Read the model definition and answer for the solid it produces. Units are mm, in the model's axes. A direction names the side the tool comes from. Coordinates: 2 decimals unless noted, no trailing zeros. Write each loop counter-clockwise with the first axis right and the second up, starting at its lowest first coordinate (ties: lowest second). Pieces come first, ordered by that corner, then holes.
(1) Given pin 1 (0.8 mm diameter, centred on x = 11, y = 5.5, fed in from +Z); pin 2 (3.5 mm diameter, centred on x = 12, z = -8, fed in from -Y); pin 3 (2 mm diameter, centred on y = 8.5, z = -11.5, fed in from +X), each flat-ended and moving along its own axis, determine where each tip first touches the part or whether it passes through.
(2) Which of the six approach directions +Z, -Z, +X, -X, +Y, -Y give full straight-line access (tool end or side, diameter ignored) to faces 3 (the cylindrical face through (17.845, 9.014, -8.921)), 4 (the flat face through (12, 6, -8)), 5 (the flat face through (5, 7, -8))?
(3) The part is cut by section C-C, the plane z = -13.25. Determine the outline of the cut face in (x, y).
(4) Determine the mould class of faces 1 (the flat face through (18, 5, -14)), 2 (the cylindrical face through (14.808, 9.699, -13.285)) for opening direction Z: pulls with the +Z half, pulls with the -Z half, needs draft (parallel to the pull), parting line crosses it, or undercut.
(5) The part is cut by section A-A, the plane x = 18.5. Determine the outline of the cut face in (y, z), and give its area (3 significant figures).
(6) The part is cut by section B-B, the plane x = 12. Determine the outline of the cut face in (y, z).
(7) The part is cut by section D-D, the plane y = 6.4. State how many separate pieces and enclosed holes the cut face has, and give its area (3 significant figures).
(8) Straight lines are drawn through the part: line 1 along Z through (x, y) = (10.5, 7.9); line 2 along Z through (x, y) = (12, 5.95); line 3 along Z through (x, y) = (18.25, 7.7). For each, find the intervals that lie inside material, in ascending order.
```python
from build123d import *

# Parameters (mm, degrees)
BOSS_EXTRUDE1_DEPTH = 10
CUT_EXTRUDE3_DEPTH  = 28.676705006
CUT_EXTRUDE6_START  = -13
CUT_EXTRUDE6_DEPTH  = 2
CUT_EXTRUDE14_START = -3
CUT_EXTRUDE14_DEPTH = 2
CUT_EXTRUDE7_START  = 10
SKETCH8_R           = 2.75
CUT_EXTRUDE7_DEPTH  = 2
CUT_EXTRUDE8_START  = -16
SKETCH10_R          = 2.25
CUT_EXTRUDE8_DEPTH  = 3
CUT_EXTRUDE9_DEPTH  = 5
SKETCH18_R          = 0.75
CUT_EXTRUDE12_DEPTH = 28.676705006
CUT_EXTRUDE13_START = 5
SKETCH19_W          = 4
SKETCH19_H          = 4
CUT_EXTRUDE13_DEPTH = 1
CUT_EXTRUDE15_START = -1
SKETCH5_R           = 1.75
CUT_EXTRUDE15_DEPTH = 2
CUT_EXTRUDE16_START = -1
CUT_EXTRUDE16_DEPTH = 2
FILLET2_R           = 0.5
FILLET3_R           = 1
POT_INSERT_DEPTH    = 2.5
POT_START           = 4
SKETCH6_R           = 2.75
POT_HOLE_DEPTH      = 1.5
SCREW_START         = 11
SKETCH14_R          = 0.8
SCREW_HOLES_DEPTH   = 9
SCREW_START_2       = 10
SKETCH15_R          = 1.25
SCREW_HEADS_DEPTH   = 2
SKETCH13_W          = 21
SKETCH13_H          = 15
CUT_EXTRUDE11_DEPTH = 5


with BuildPart() as part:
    # Sketch1 → Boss-Extrude1 (new body)
    with BuildSketch(Plane(origin=(0, 0, 0), x_dir=(1, 0, 0), z_dir=(0, 1, 0))):
        with BuildLine():
            Line((21, 15), (21, 8))
            Line((21, 8), (21, 1))
            Line((21, 1), (12, 1))
            Line((12, 1), (2.253205655, 1))
            ThreePointArc((2.253205655, 1), (0, 8), (2.253205655, 15))
            Line((2.253205655, 15), (12, 15))
            Line((12, 15), (21, 15))
        make_face()
    extrude(amount=BOSS_EXTRUDE1_DEPTH)

    # Sketch4 → Cut-Extrude3 (cut, through all)
    with BuildSketch(Plane.XY):
        with BuildLine():
            Line((21, 14), (12, 14))
            ThreePointArc((12, 14), (18.363961031, 11.363961031), (21, 5))
            Line((21, 5), (21, 14))
        make_face()
        with BuildLine():
            Line((21, -4), (21, 5))
            ThreePointArc((21, 5), (18.363961031, -1.363961031), (12, -4))
            Line((12, -4), (21, -4))
        make_face()
    extrude(amount=-CUT_EXTRUDE3_DEPTH, mode=Mode.SUBTRACT)

    # Sketch7 → Cut-Extrude6 (cut)
    with BuildSketch(Plane.XY.offset(CUT_EXTRUDE6_START)):
        Polygon((21, 5.5), (21, 11), (10, 11), (10, 7.5), (0, 7.5), (0, 3.5), (21, 3.5), align=None)
    extrude(amount=CUT_EXTRUDE6_DEPTH, mode=Mode.SUBTRACT)

    # Sketch21 → Cut-Extrude14 (cut)
    with BuildSketch(Plane.XY.offset(CUT_EXTRUDE14_START)):
        Polygon((21, 5.5), (21, 11), (10, 11), (10, 7.5), (0, 7.5), (0, 3.5), (21, 3.5), align=None)
    extrude(amount=-CUT_EXTRUDE14_DEPTH, mode=Mode.SUBTRACT)

    # Sketch8 → Cut-Extrude7 (cut)
    with BuildSketch(Plane(origin=(0, 0, 0), x_dir=(1, 0, 0), z_dir=(0, 1, 0)).offset(CUT_EXTRUDE7_START)):
        with Locations(Location((12, 8, 0), (0, 0, 270))):
            Circle(SKETCH8_R)
    extrude(amount=-CUT_EXTRUDE7_DEPTH, mode=Mode.SUBTRACT)

    # Sketch10 → Cut-Extrude8 (cut)
    with BuildSketch(Plane.XY.offset(CUT_EXTRUDE8_START)):
        with Locations(Location((12, 5, 0), (0, 0, 221.810314896))):
            Circle(SKETCH10_R)
    extrude(amount=CUT_EXTRUDE8_DEPTH, mode=Mode.SUBTRACT)

    # Sketch11 → Cut-Extrude9 (cut)
    with BuildSketch(Plane(origin=(0, 0, 0), x_dir=(0, 0, -1), z_dir=(1, 0, 0))):
        Polygon((8, 2), (13, 2), (13, 8), (3, 8), (3, 2), align=None)
    extrude(amount=CUT_EXTRUDE9_DEPTH, mode=Mode.SUBTRACT)

    # Sketch18 → Cut-Extrude12 (cut, through all)
    with BuildSketch(Plane.XY):
        with Locations((12, 5)):
            Circle(SKETCH18_R)
    extrude(amount=-CUT_EXTRUDE12_DEPTH, mode=Mode.SUBTRACT)

    # Sketch19 → Cut-Extrude13 (cut, symmetric)
    with BuildSketch(Plane(origin=(0, 0, 0), x_dir=(1, 0, 0), z_dir=(0, 1, 0)).offset(CUT_EXTRUDE13_START)):
        with Locations((12, 8)):
            Rectangle(SKETCH19_W, SKETCH19_H)
    extrude(amount=CUT_EXTRUDE13_DEPTH, both=True, mode=Mode.SUBTRACT)

    # Sketch5 → Cut-Extrude15 (cut)
    with BuildSketch(Plane.XY.offset(CUT_EXTRUDE15_START)):
        with Locations((12, 5)):
            Circle(SKETCH5_R)
    extrude(amount=-CUT_EXTRUDE15_DEPTH, mode=Mode.SUBTRACT)

    # Sketch26 → Cut-Extrude16 (cut)
    with BuildSketch(Plane.XY.offset(CUT_EXTRUDE16_START)):
        with BuildLine():
            Line((16.483314774, 10), (19.483314774, 10))
            ThreePointArc((19.483314774, 10), (20.800790614, 6.883105034), (20.874119675, 3.5))
            Line((20.874119675, 3.5), (17.874119675, 3.5))
            ThreePointArc((17.874119675, 3.5), (17.800790614, 6.883105034), (16.483314774, 10))
        make_face()
    extrude(amount=-CUT_EXTRUDE16_DEPTH, mode=Mode.SUBTRACT)

    # Fillet2
    fillet2_edges = [part.edges().sort_by_distance(p)[0] for p in [
        (12, 8, -10.75),
    ]]
    fillet(fillet2_edges, radius=FILLET2_R)

    # Fillet3
    # the kernel refuses this fillet: 1 mm, written as the material it takes off along each edge
    with BuildSketch(Plane(origin=(12, 5, -13), x_dir=(0.6472427025312245, 0.7622839917118008, 0), z_dir=(-0.7622839917118008, 0.6472427025312245, 0))) as fillet3_piece_1_section:
        with BuildLine():
            CenterArc((9 - FILLET3_R, FILLET3_R), FILLET3_R, 270, 90)
            Line((9 - FILLET3_R, 0), (9, 0))
            Line((9, 0), (9, FILLET3_R))
        make_face()
    fillet3_piece_1 = revolve(axis=Axis((12, 5, -13), (0, 0, -1)), revolution_arc=75.177010416, mode=Mode.PRIVATE)
    fillet3_piece_1 = split(fillet3_piece_1, bisect_by=Plane(origin=(20.22008164, 3.5, -13.28352735), z_dir=(0, 1, 0)), keep=Keep.TOP, mode=Mode.PRIVATE)
    add(fillet3_piece_1, mode=Mode.SUBTRACT)
    with BuildSketch(Plane(origin=(12, 5, -11), x_dir=(0.9025022770828605, -0.43068508200337235, 0), z_dir=(-0.43068508200337235, -0.9025022770828605, 0))) as fillet3_piece_2_section:
        with BuildLine():
            CenterArc((9 - FILLET3_R, FILLET3_R), FILLET3_R, 270, 90)
            Line((9 - FILLET3_R, 0), (9, 0))
            Line((9, 0), (9, FILLET3_R))
        make_face()
    fillet3_piece_2 = revolve(axis=Axis((12, 5, -11), (0, 0, 1)), revolution_arc=75.177010416, mode=Mode.PRIVATE)
    fillet3_piece_2 = split(fillet3_piece_2, bisect_by=Plane(origin=(20.220081643, 3.5, -10.716472653), z_dir=(0, 1, 0)), keep=Keep.TOP, mode=Mode.PRIVATE)
    add(fillet3_piece_2, mode=Mode.SUBTRACT)
    with BuildSketch(Plane(origin=(21.983314774, 10, -11), x_dir=(0, 0, 1), z_dir=(-1, 0, 0))) as fillet3_piece_3:
        with BuildLine():
            CenterArc((FILLET3_R, -FILLET3_R), FILLET3_R, 90, 90)
            Line((0, -FILLET3_R), (0, 0))
            Line((0, 0), (FILLET3_R, 0))
        make_face()
    extrude(amount=11.983314774, mode=Mode.SUBTRACT)
    with BuildSketch(Plane(origin=(21.983314774, 10, -13), x_dir=(0, 0, -1), z_dir=(-1, 0, 0))) as fillet3_piece_4:
        with BuildLine():
            CenterArc((FILLET3_R, FILLET3_R), FILLET3_R, 180, 90)
            Line((0, FILLET3_R), (0, 0))
            Line((0, 0), (FILLET3_R, 0))
        make_face()
    extrude(amount=11.983314774, mode=Mode.SUBTRACT)

    # Sketch3 → Pot Insert (cut)
    with BuildSketch(Plane(origin=(28.28760271, 0, 0), x_dir=(1, 0, 0), z_dir=(0, 1, 0))):
        Polygon((-25.28760271, 12.5), (-20.53760271, 12.5), (-20.53760271, 13.5), (-16.28760271, 13.5), (-12.291072924, 13.5), (-12.291072924, 12.500096395), (-10.791072924, 9.500096395), (-9.28760271, 9.500096395), (-9.28760271, 8), (-9.28760271, 6.5), (-10.78760271, 6.5), (-12.28760271, 3.5), (-12.28760271, 2.5), (-16.28760271, 2.5), (-20.53760271, 2.5), (-20.53760271, 3.5), (-25.28760271, 3.5), (-25.28760271, 8), align=None)
    extrude(amount=POT_INSERT_DEPTH, mode=Mode.SUBTRACT)

    # Sketch6 → Pot Hole (cut)
    with BuildSketch(Plane(origin=(0, 0, 0), x_dir=(1, 0, 0), z_dir=(0, 1, 0)).offset(POT_START)):
        with Locations(Location((12, 8, 0), (0, 0, 270))):
            Circle(SKETCH6_R)
    extrude(amount=-POT_HOLE_DEPTH, mode=Mode.SUBTRACT)

    # Sketch14 → Screw Holes (cut)
    with BuildSketch(Plane(origin=(0, 0, 0), x_dir=(1, 0, 0), z_dir=(0, 1, 0)).offset(SCREW_START)):
        with Locations(Location((7, 8, 0), (0, 0, 270))):
            Circle(SKETCH14_R)
        with Locations(Location((17, 8, 0), (0, 0, 270))):
            Circle(SKETCH14_R)
    extrude(amount=-SCREW_HOLES_DEPTH, mode=Mode.SUBTRACT)

    # Sketch15 → Screw Heads (cut)
    with BuildSketch(Plane(origin=(0, 0, 0), x_dir=(1, 0, 0), z_dir=(0, 1, 0)).offset(SCREW_START_2)):
        with Locations(Location((7, 8, 0), (0, 0, 270))):
            Circle(SKETCH15_R)
        with Locations(Location((17, 8, 0), (0, 0, 270))):
            Circle(SKETCH15_R)
    extrude(amount=-SCREW_HEADS_DEPTH, mode=Mode.SUBTRACT)

    # Sketch13 → Cut-Extrude11 (cut)
    with BuildSketch(Plane(origin=(0, 0, 0), x_dir=(1, 0, 0), z_dir=(0, 1, 0))):
        with Locations((10.5, 7.5)):
            Rectangle(SKETCH13_W, SKETCH13_H)
    extrude(amount=CUT_EXTRUDE11_DEPTH, mode=Mode.SUBTRACT)


solid = part.part
```
Computed:
1. pin 1: stops at z = -5
1. pin 2: stops at y = 6
1. pin 3: stops at x = 20.25
2. face 3: +Y
2. face 4: -Y
2. face 5: -X, -Y
3. outline: (1.21, 5) - (9.75, 5) arc R2.25 cw to (14.25, 5) - (20.66, 5) arc R8.66 ccw to (19.3, 9.66) - (10, 9.66) - (10, 10) - (1.21, 10) - close
4. face 1: needs draft
4. face 2: undercut
5. outline: (5, -15) - (10, -15) - (10, -14) arc R1 ccw to (9, -13) - (5, -13) - close; (5, -11) - (9, -11) arc R1 ccw to (10, -10) - (10, -5) - (5, -5) - close
5. area: 39.6 mm2
6. outline: (5.75, -11) - (9, -11) arc R1 ccw to (9.66, -10.75) - (8.5, -10.75) arc R0.5 cw to (8, -10.25) - (8, -5.75) arc R0.5 cw to (8.5, -5.25) - (10, -5.25) - (10, -5) - (5.75, -5) - (5.75, -6) - (6, -6) - (6, -10) - (5.75, -10) - close; (6.75, -3) - (10, -3) - (10, -1) - (6.75, -1) - close; (7.25, -15) - (10, -15) - (10, -14) arc R1 ccw to (9, -13) - (7.25, -13) - close
7. separate pieces: 5
7. enclosed holes: 2
7. area: 151 mm2
8. line 1: z = -15 to -13, -11 to -5, -3 to -1
8. line 2: z = -11 to -10, -6 to -5
8. line 3: z = -15 to -13, -11 to -5
